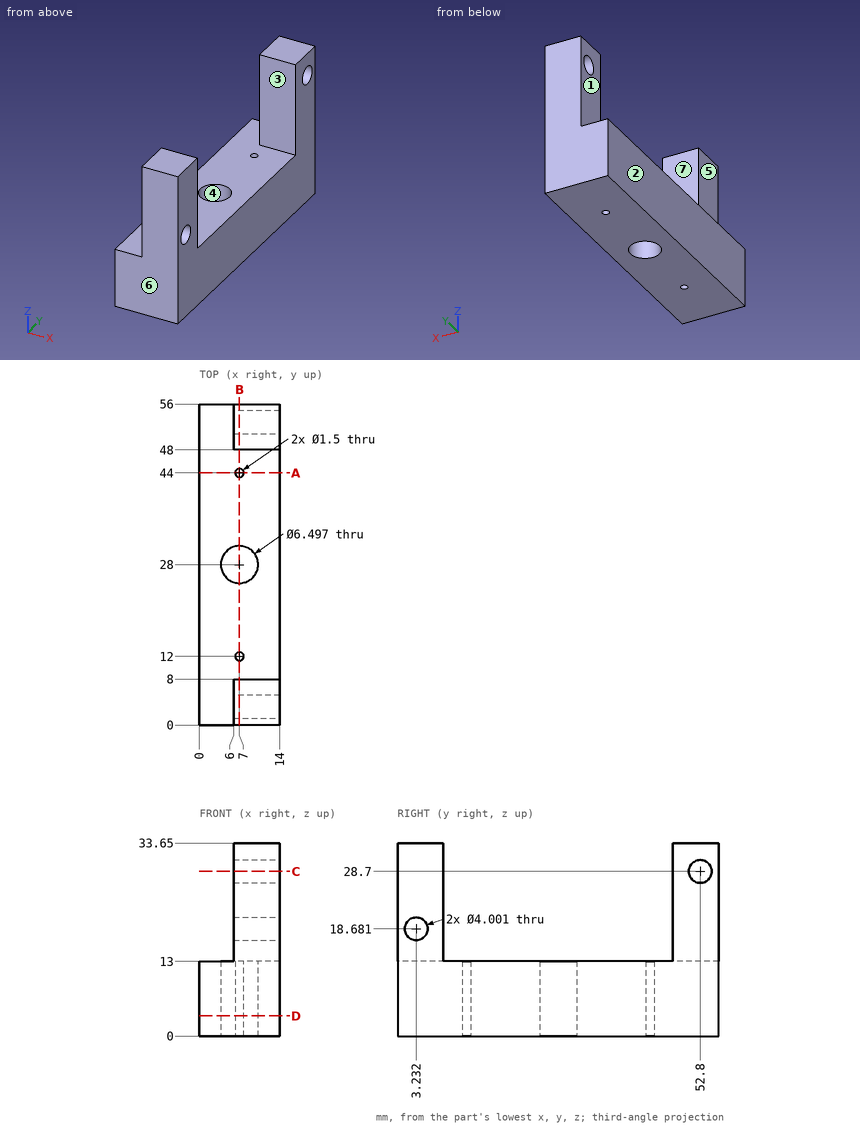
Source: three-view drawing plus pictorial views. Frame: mm from the lowest corner of the part. A direction names the side the tool comes from. Round coordinates to 2 decimals unless told otherwise and drop trailing zeros. Loops run counter-clockwise (first coordinate to the right, second up) from the corner with the lowest first, then second, coordinate; pieces in that order, holes last. Notation, with made-up numbers: (66.5, 82.25) -> (105.5, 82.25) arc R32 ccw to (105.5, 115.25) -> close; hole circle Ø4 at (-29.5, 27.5). An arc over 180 degrees is marked (long way). Use one line per item in the form item = value.
Item 1: Cut plane D-D on z = 3.5. Output: boundary loops of the cut face in (x, y), then the cut area to 3 significant figures.
Evaluation:
outline = (0, 0) -> (14, 0) -> (14, 56) -> (0, 56) -> close; hole circle Ø6.5 at (7, 28); hole circle Ø1.5 at (7, 12); hole circle Ø1.5 at (7, 44)
area = 747 mm2
Item 2: Cut plane B-B on x = 7. Output: boundary loops of the cut face in (y, z).
Evaluation:
outline = (0, 0) -> (11.25, 0) -> (11.25, 13) -> (8, 13) -> (8, 33.65) -> (0, 33.65) -> close; (12.75, 0) -> (24.75, 0) -> (24.75, 13) -> (12.75, 13) -> close; (31.25, 0) -> (43.25, 0) -> (43.25, 13) -> (31.25, 13) -> close; (44.75, 0) -> (56, 0) -> (56, 33.65) -> (48, 33.65) -> (48, 13) -> (44.75, 13) -> close; hole circle Ø4 at (3.23, 18.68); hole circle Ø4 at (52.8, 28.7)
Item 3: Cut plane C-C on z = 28.7. Output: boundary loops of the cut face in (x, y).
Evaluation:
outline = (6, 0) -> (14, 0) -> (14, 8) -> (6, 8) -> close; (6, 48) -> (14, 48) -> (14, 50.8) -> (6, 50.8) -> close; (6, 54.8) -> (14, 54.8) -> (14, 56) -> (6, 56) -> close
Item 4: Access query for the marked faces 1, 2 and 3. Directions: +Z, -Z, +X, -X, +Y, -Y. A direction counts if a zero-diameter tool reaches every point of the face in a straight line with its end or side. Return the directions, or none.
Evaluation:
face_1 = +Z, -X, +Y, -Y
face_2 = +Z, -Z, -X, +Y, -Y
face_3 = +Z, +X, -X
Item 5: Draft query along Y for the marked faces 4, 5, 6 and 7. Return one class per face: released by +Y, released by -Y, zero draft, split by the parting line, or undercut.
Evaluation:
face_4 = undercut
face_5 = zero draft
face_6 = released by -Y
face_7 = undercut
Item 6: Material intervals for probe 1 along Y at (x, z) = (7, 8.5); probe 2 along Z at (x, y) = (11.25, 52.8); probe 3 along Y at (x, z) = (7.5, 28.7), sorted ascending.
Evaluation:
probe_1 = 0 to 11.25, 12.75 to 24.75, 31.25 to 43.25, 44.75 to 56
probe_2 = 0 to 26.7, 30.7 to 33.65
probe_3 = 0 to 8, 48 to 50.8, 54.8 to 56
Item 7: Cut plane A-A on y = 44. Output: boundary loops of the cut face in (x, z).
Evaluation:
outline = (0, 0) -> (6.25, 0) -> (6.25, 13) -> (0, 13) -> close; (7.75, 0) -> (14, 0) -> (14, 13) -> (7.75, 13) -> close
Item 8: Contact query for flat-ended pins moving along their axis: pin 1 Ø4 at (x, y) = (3.5, 7) entering from +Z; pin 2 Ø5 at (x, y) = (7, 28) entering from -Z; pin 3 Ø4 at (y, z) = (3, 19) entering from -X. Output: stop coordinate, or through.
Evaluation:
pin_1 = 13
pin_2 = through
pin_3 = 6
